Check sheet for the modelled part. Datum: model origin and axes. Units: mm. A direction names the side the tool comes from. Round coordinates to 2 decimals unless told otherwise and drop trailing zeros. Order: outer loops, then holes, each group sorted by start corner. A loop starts at its lowest first (then second) coordinate and runs counter-clockwise, first axis right, second up.
Q1. Cross-section at C-C on z = 17.5. Record the cut outline in (x, y).
Q2. Cross-section at D-D on z = 23.25. Record the cut outline in (x, y).
Q3. Cross-section at B-B on x = 45.5. Record the cut outline in (y, z).
Q4. Depth check by flat-ended pin: P1, Ø8, axis at x = 55, y = 7, coming from the +Z side; P2, Ø3, axis at x = 5, z = 11, coming from the +Y side; P3, Ø24, axis at x = 24, y = 39.5, coming from the -Z side; P4, Ø1, axis at y = 11.5, z = 21, coming from the +X side. Enter the tip coordinate at first touch or a pass-through.
Q5. Mould release check, pull along X, two halves, no side actions. Record for faces 1 (the flat face through (20, 0, 10)), 2 (the cylindrical face through (65, 44.604, 22.465)), 3 (the flat face through (10, 7, -2)): +X half, -X half, draft (parallel to the pull), parting line (faces both ways), or undercut.
Q6. Set-up check for faces 4 (the flat face through (22.381, 36, 22)), 5 (the flat face through (25, 34, 0)), 6 (the flat face through (53, 43, 20)): record each of +Z, -Z, +X, -X, +Y, -Y from which the full face is reachable in a straight line by a thin tool's end or side.
Q7. Cross-section at A-A on y = 8. Record the cut outline in (x, z).
Q8. Scan lines: probe 1 along Y at (x, z) = (55, -2.9); probe 2 along Y at (x, z) = (69, 21.5); probe 3 along Z at (x, y) = (58, 38.5). Record each from-to range of solid material in increasing order.
from build123d import *

# Parameters (mm, degrees)
DODANIE_WYCI_GNI_CIE1_DEPTH = 20
SZKIC2_R                    = 3.5
DODANIE_WYCI_GNI_CIE2_DEPTH = 5
SZKIC3_R                    = 3
DODANIE_WYCI_GNI_CIE3_DEPTH = 5


with BuildPart() as part:
    # Szkic1 → Dodanie-wyciągnięcie1 (new body)
    with BuildSketch(Plane.XY):
        Polygon((0, 0), (40, 0), (40, 52.681400645), (22.380650018, 52.681400645), (10, 35), (10, 14), (0, 14), align=None)
    extrude(amount=DODANIE_WYCI_GNI_CIE1_DEPTH)

    # Szkic2 → Dodanie-wyciągnięcie2 (add)
    with BuildSketch(Plane(origin=(0, 0, 0), x_dir=(-1, 0, 0), z_dir=(0, 0, -1))):
        with BuildLine():
            Line((-10, 0), (-10, 14))
            Line((-10, 14), (-54.922294035, 14))
            ThreePointArc((-54.922294035, 14), (-62, 7.00043131), (-54.922294026, 0.000862629))
            Line((-54.922294026, 0.000862629), (-10, 0))
        make_face()
        with Locations((-55, 7.000431315)):
            Circle(SZKIC2_R, mode=Mode.SUBTRACT)
    extrude(amount=DODANIE_WYCI_GNI_CIE2_DEPTH)

    # Szkic3 → Dodanie-wyciągnięcie3 (add)
    with BuildSketch(Plane.XY.offset(20)):
        with BuildLine():
            Line((22.380650018, 52.681400645), (22.380650018, 18.546912235))
            Line((22.380650018, 18.546912235), (70.022924699, 40.762869771))
            ThreePointArc((70.022924699, 40.762869771), (73.484603525, 47.782460025), (67.380650018, 52.681400645))
            Line((67.380650018, 52.681400645), (22.380650018, 52.681400645))
        make_face()
        with Locations((67.380650018, 46.429246111)):
            Circle(SZKIC3_R, mode=Mode.SUBTRACT)
    extrude(amount=DODANIE_WYCI_GNI_CIE3_DEPTH)


solid = part.part
Results found:
1. outline: (0, 0) - (40, 0) - (40, 52.68) - (22.38, 52.68) - (10, 35) - (10, 14) - (0, 14) - close
2. outline: (22.38, 18.55) - (70.02, 40.76) arc R6.25 ccw to (67.38, 52.68) - (22.38, 52.68) - close; hole circle Ø6 at (67.38, 46.43)
3. outline: (0, -5) - (14, -5) - (14, 0) - (0, 0) - close; (29.33, 20) - (52.68, 20) - (52.68, 25) - (29.33, 25) - close
4. P1: stops at z = 0
4. P2: stops at y = 14
4. P3: stops at z = 0
4. P4: passes through
5. face 1: draft
5. face 2: undercut
5. face 3: -X half
6. face 4: +Z, -X, +Y, -Y
6. face 5: -Z, +X, -X, +Y
6. face 6: -Z, +X, +Y, -Y
7. outline: (0, 0) - (10, 0) - (10, -5) - (51.65, -5) - (51.65, 0) - (40, 0) - (40, 20) - (0, 20) - close; (58.35, -5) - (61.93, -5) - (61.93, 0) - (58.35, 0) - close
8. probe 1: y = 0 to 3.5, 10.5 to 14
8. probe 2: y = 40.29 to 43.9, 48.95 to 52.47
8. probe 3: z = 20 to 25
